Check sheet for the modelled part. Datum: model origin and axes. Units: mm. Face numbers are marked on the shaded views. A direction names the side the tool comes from. Round coordinates to 2 decimals unless told otherwise and drop trailing zeros. Order: outer loops, then holes, each group sorted by start corner. A loop starts at its lowest first (then second) coordinate and runs counter-clockwise, first axis right, second up. Notation, with made-up numbers: (25.5, -19.5) -> (29.5, -19.5) arc R30 ccw to (29.5, 13.5) -> close; hole circle Ø3 at (-8.5, 11). An arc over 180 degrees is marked (long way). Answer in a Markdown table with one row per item.
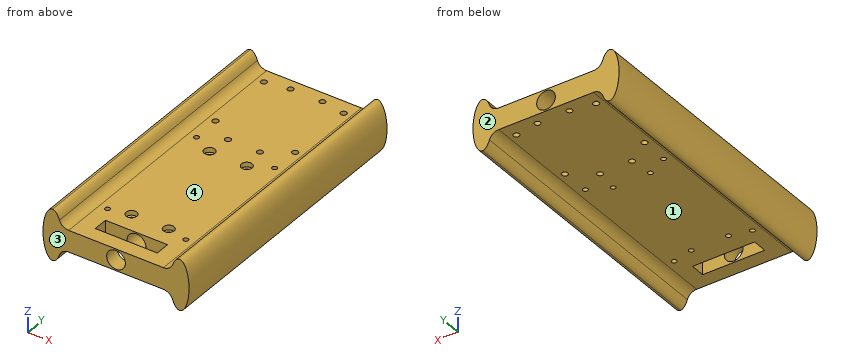
```python
from build123d import *

# Parameters (mm, degrees)
SKETCH1_RX                        = 13
SKETCH1_RY                        = 4.85
SKETCH1_W                         = 65
SKETCH1_H                         = 11
SKETCH1_R                         = 4.7775
BOSS_EXTRUDE1_DEPTH               = 145
FILLET1_R                         = 5
SKETCH3_W                         = 31.75
SKETCH3_H                         = 7.5
CUT_EXTRUDE2_DEPTH                = 8.5000001
CUT_EXTRUDE2_DEPTH_BACK           = 19.5000001
TAP_DRILL_FOR_M3X0_5_TAP1_D       = 2.5
SKETCH6_R                         = 2.75
CUT_EXTRUDE4_DEPTH                = 2.4
TAP_DRILL_FOR_M3_TAP1_D           = 2.5
TAP_DRILL_FOR_M3_TAP1_CSINK_D     = 2.55
TAP_DRILL_FOR_M3_TAP1_CSINK_ANGLE = 90
SKETCH9_R                         = 1.5
CUT_EXTRUDE5_DEPTH                = 19.5000001
CUT_EXTRUDE6_REACH                = 20.5
SKETCH5_R                         = 1.525


with BuildPart() as part:
    # Sketch1 → Boss-Extrude1 (new body)
    with BuildSketch(Plane(origin=(0, 0, 0), x_dir=(1, 0, 0), z_dir=(0, 1, 0))):
        with Locations(Location((-32.5, 0), (0, 0, -90))):
            Ellipse(SKETCH1_RX, SKETCH1_RY)
        with Locations(Location((32.5, 0), (0, 0, 90))):
            Ellipse(SKETCH1_RX, SKETCH1_RY)
        Rectangle(SKETCH1_W, SKETCH1_H)
        Circle(SKETCH1_R, mode=Mode.SUBTRACT)
    extrude(amount=BOSS_EXTRUDE1_DEPTH)

    # Fillet1
    fillet1_edges = [part.edges().sort_by_distance(p)[0] for p in [
        (-28.105445223, 72.5, -5.5),
        (28.105445223, 72.5, -5.5),
        (28.105445223, 72.5, 5.5),
        (-28.105445223, 72.5, 5.5),
    ]]
    fillet(fillet1_edges, radius=FILLET1_R)

    # Sketch3 → Cut-Extrude2 (cut, two sides)
    with BuildSketch(Plane(origin=(0, 0, -5.5), x_dir=(-1, 0, 0), z_dir=(0, 0, -1))) as cut_extrude2_sk:
        with Locations((0, 11.25)):
            Rectangle(SKETCH3_W, SKETCH3_H)
    extrude(amount=CUT_EXTRUDE2_DEPTH, mode=Mode.SUBTRACT)
    extrude(cut_extrude2_sk.sketch, amount=-CUT_EXTRUDE2_DEPTH_BACK, mode=Mode.SUBTRACT)

    # Tap Drill for M3x0.5 Tap1 (through all)
    with Locations(Plane(origin=(9.525, 82.15, -5.5), x_dir=(-1, 0, 0), z_dir=(0, 0, -1))):
        with Locations((0, 0), (19.05, 0), (19.05, -57.15), (0, -57.15)):
            Hole(TAP_DRILL_FOR_M3X0_5_TAP1_D / 2)

    # Sketch6 → Cut-Extrude4 (cut)
    with BuildSketch(Plane.XY.offset(5.5)):
        with Locations((9.525, 82.15)):
            Circle(SKETCH6_R)
        with Locations((-9.525, 82.15)):
            Circle(SKETCH6_R)
        with Locations((9.525, 25)):
            Circle(SKETCH6_R)
        with Locations((-9.525, 25)):
            Circle(SKETCH6_R)
    extrude(amount=-CUT_EXTRUDE4_DEPTH, mode=Mode.SUBTRACT)

    # Tap Drill for M3 Tap1 (through all)
    with Locations(Plane.XY.offset(5.5)):
        with Locations((-20, 87.5), (20, 87.5), (20, 22.5), (-20, 22.5)):
            CounterSinkHole(TAP_DRILL_FOR_M3_TAP1_D / 2, TAP_DRILL_FOR_M3_TAP1_CSINK_D / 2, counter_sink_angle=TAP_DRILL_FOR_M3_TAP1_CSINK_ANGLE)

    # Sketch9 → Cut-Extrude5 (cut, through all)
    with BuildSketch(Plane(origin=(0, 0, -5.5), x_dir=(-1, 0, 0), z_dir=(0, 0, -1))):
        with Locations((-8.168, 139.5)):
            Circle(SKETCH9_R)
        with Locations((8.168, 139.5)):
            Circle(SKETCH9_R)
        with Locations((8.168, 93.7)):
            Circle(SKETCH9_R)
        with Locations((-8.168, 93.7)):
            Circle(SKETCH9_R)
    extrude(amount=-CUT_EXTRUDE5_DEPTH, mode=Mode.SUBTRACT)

    # Sketch5 → Cut-Extrude6 (cut, up to next)
    with BuildSketch(Plane.XY.offset(5.5), mode=Mode.PRIVATE) as cut_extrude6_sk1:
        with Locations((20.4, 102)):
            Circle(SKETCH5_R)
    cut_extrude6_tool1 = extrude(cut_extrude6_sk1.sketch, amount=-CUT_EXTRUDE6_REACH, mode=Mode.PRIVATE) & part.part
    add(cut_extrude6_tool1.solids().sort_by_distance((20.4, 102, 5.5))[0], mode=Mode.SUBTRACT)
    # Sketch5 → Cut-Extrude6 (cut, up to next)
    with BuildSketch(Plane.XY.offset(5.5), mode=Mode.PRIVATE) as cut_extrude6_sk2:
        with Locations((-20.4, 102)):
            Circle(SKETCH5_R)
    cut_extrude6_tool2 = extrude(cut_extrude6_sk2.sketch, amount=-CUT_EXTRUDE6_REACH, mode=Mode.PRIVATE) & part.part
    add(cut_extrude6_tool2.solids().sort_by_distance((-20.4, 102, 5.5))[0], mode=Mode.SUBTRACT)
    # Sketch5 → Cut-Extrude6 (cut, up to next)
    with BuildSketch(Plane.XY.offset(5.5), mode=Mode.PRIVATE) as cut_extrude6_sk3:
        with Locations((20.4, 137.5)):
            Circle(SKETCH5_R)
    cut_extrude6_tool3 = extrude(cut_extrude6_sk3.sketch, amount=-CUT_EXTRUDE6_REACH, mode=Mode.PRIVATE) & part.part
    add(cut_extrude6_tool3.solids().sort_by_distance((20.4, 137.5, 5.5))[0], mode=Mode.SUBTRACT)
    # Sketch5 → Cut-Extrude6 (cut, up to next)
    with BuildSketch(Plane.XY.offset(5.5), mode=Mode.PRIVATE) as cut_extrude6_sk4:
        with Locations((-20.4, 137.5)):
            Circle(SKETCH5_R)
    cut_extrude6_tool4 = extrude(cut_extrude6_sk4.sketch, amount=-CUT_EXTRUDE6_REACH, mode=Mode.PRIVATE) & part.part
    add(cut_extrude6_tool4.solids().sort_by_distance((-20.4, 137.5, 5.5))[0], mode=Mode.SUBTRACT)


solid = part.part
```
(1) Tool access check on the marked faces 1 and 2. Record the directions out of +Z, -Z, +X, -X, +Y, -Y that give a thin tool (end or side, any length) a straight path to the whole face; none if there is none.
Solutions:
| item | result |
|---|---|
| face 1 | -Z, +Y, -Y |
| face 2 | +Z, -Z, +X, -X, +Y |
(2) Depth check by flat-ended pin: pin 1 Ø3 at (x, y) = (-9.5, 81) entering from +Z; pin 2 Ø5 at (x, y) = (8.168, 139.5) entering from -Z; pin 3 Ø3 at (x, y) = (-10.5, 96.5) entering from +Z. Enter the tip coordinate at first touch or a pass-through.
Solutions:
| item | result |
|---|---|
| pin 1 | z = 3.1 |
| pin 2 | z = -5.5 |
| pin 3 | z = 5.5 |
(3) Draft check along X on the marked faces 3 and 4. Enter one of: pulls with the +X half, pulls with the -X half, needs draft (parallel to the pull), parting line crosses it, or undercut.
Solutions:
| item | result |
|---|---|
| face 3 | needs draft |
| face 4 | undercut |
(4) Section check A-A on x = -14. Record the boundary of the cut face in (y, z).
Solutions:
| item | result |
|---|---|
| outline | (0, -5.5) -> (7.5, -5.5) -> (7.5, 5.5) -> (0, 5.5) -> close; (15, -5.5) -> (145, -5.5) -> (145, 5.5) -> (15, 5.5) -> close |
(5) Scan lines: probe 1 along Y at (x, z) = (-12, -3.25); probe 2 along X at (y, z) = (5.25, 0); probe 3 along Z at (x, y) = (0, 103). Record each from-to range of solid material in increasing order. Write a range as from..to.
Solutions:
| item | result |
|---|---|
| probe 1 | 0..7.5, 15..145 |
| probe 2 | -37.35..-4.78, 4.78..37.35 |
| probe 3 | -5.5..-4.78, 4.78..5.5 |
(6) Section check B-B on x = 0. Record the boundary of the cut face in (y, z), plus the area to 3 significant figures.
Solutions:
| item | result |
|---|---|
| outline | (0, -5.5) -> (7.5, -5.5) -> (7.5, -4.78) -> (0, -4.78) -> close; (0, 4.78) -> (7.5, 4.78) -> (7.5, 5.5) -> (0, 5.5) -> close; (15, -5.5) -> (145, -5.5) -> (145, -4.78) -> (15, -4.78) -> close; (15, 4.78) -> (145, 4.78) -> (145, 5.5) -> (15, 5.5) -> close |
| area | 199 mm^2 |
(7) Section check C-C on y = 93.7. Give the number of separate pieces and of enclosed holes in the cut face, plus the area to 3 significant figures.
Solutions:
| item | result |
|---|---|
| separate pieces | 3 |
| enclosed holes | 1 |
| area | 881 mm^2 |
